For this review, use the dimensioned drawing (mm, ordinates from the lowest corner) and the shaded views. A direction names the side the tool comes from. Give positions to 0.01 mm unless a question says otherwise; leave off trailing zeros. Order: outer loops, then holes, each group sorted by start corner. A loop starts at its lowest first (then second) coordinate and runs counter-clockwise, first axis right, second up.
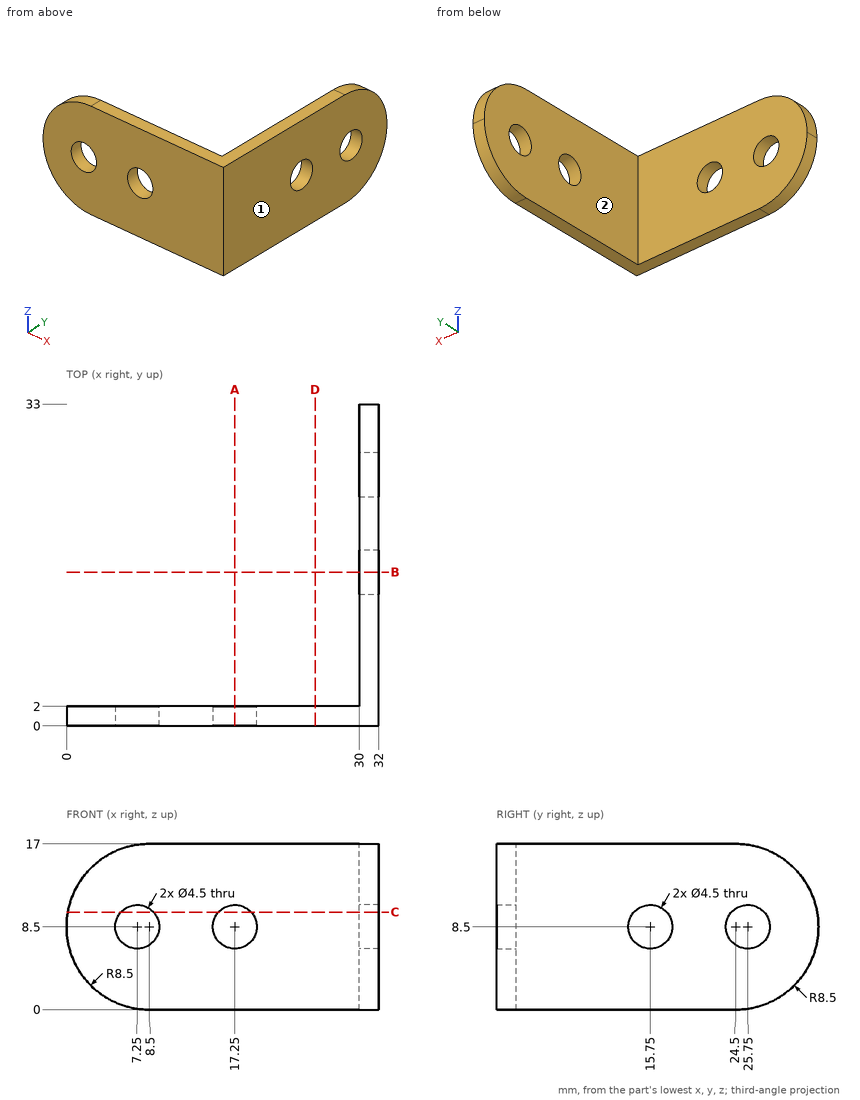
1. Take a section at A-A (x = 17.25). State the section outline as (y, z) points.
Recorded:
outline: (0, 0) - (2, 0) - (2, 6.25) - (0, 6.25) - close; (0, 10.75) - (2, 10.75) - (2, 17) - (0, 17) - close
2. Take a section at B-B (y = 15.75). State the section outline as (x, z) points, then the cut area to 3 significant figures.
Recorded:
outline: (30, 0) - (32, 0) - (32, 6.25) - (30, 6.25) - close; (30, 10.75) - (32, 10.75) - (32, 17) - (30, 17) - close
area: 25.0 mm2
3. Take a section at C-C (z = 10). State the section outline as (x, y) points, then the cut area to 3 significant figures.
Recorded:
outline: (0.13, 0) - (5.57, 0) - (5.57, 2) - (0.13, 2) - close; (8.93, 0) - (15.57, 0) - (15.57, 2) - (8.93, 2) - close; (18.93, 0) - (32, 0) - (32, 14.07) - (30, 14.07) - (30, 2) - (18.93, 2) - close; (30, 17.43) - (32, 17.43) - (32, 24.07) - (30, 24.07) - close; (30, 27.43) - (32, 27.43) - (32, 32.87) - (30, 32.87) - close
area: 98.6 mm2
4. For pin 1 (5 mm diameter, centred on y = 24.5, z = 4.5, fed in from -X); pin 2 (6 mm diameter, centred on x = 7.25, z = 8.5, fed in from +Y), all flat-tipped, find the tip position at first contact; note any pin that passes through.
Recorded:
pin 1: stops at x = 30
pin 2: stops at y = 2
5. For line 1 along Y through (x, z) = (15, 12); line 2 along Z through (x, y) = (31.4, 15.75); line 3 along X through (y, z) = (16, 2), list the stretches that pass through material, from the lowest coordinate up.
Recorded:
line 1: y = 0 to 2
line 2: z = 0 to 6.25, 10.75 to 17
line 3: x = 30 to 32
6. Machinability: for the marked faces 1 and 2, which of the approach directions +Z, -Z, +X, -X, +Y, -Y give a long, thin tool a straight path to every point of the face, cutting with its end or side? Answer none if there is none.
Recorded:
face 1: +Z, -Z, +X, +Y, -Y
face 2: +Z, -Z, -X, +Y
7. Take a section at D-D (x = 25.5). State the section outline as (y, z) points.
Recorded:
outline: (0, 0) - (2, 0) - (2, 17) - (0, 17) - close
